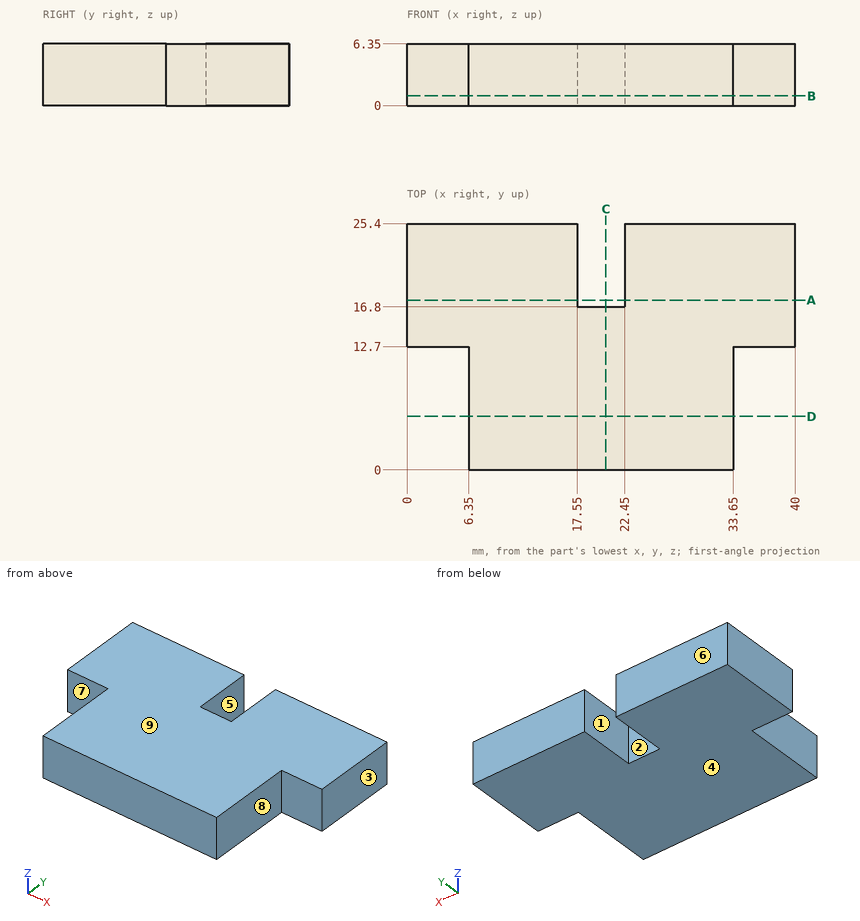
Part print with two shaded views. Sizes in mm from the minimum x, y, z corner. A direction names the side the tool comes from. Coordinates: 2 decimals unless noted, no trailing zeros. Order: outer loops, then holes, each group sorted by start corner. A loop starts at its lowest first (then second) coordinate and runs counter-clockwise, first axis right, second up. Notation, with made-up numbers: (-16, -4.75) - (2, -4.75) arc R20 ccw to (2, 22.25) - close; hole circle Ø1 at (31, 81). An arc over 180 degrees is marked (long way). Write item = value, one per line. Start each with the question number.
1) Saw through at A-A on y = 17.5. Write the cut outline in (x, z), then the cut area to 3 significant figures.
2) Wall check: line 1 along X through (y, z) = (19.75, 4.5); line 2 along Y through (x, z) = (6, 6.25); line 3 along X through (y, z) = (6, 3.5). Give the ranges that are in metal, low to high. Write a range as from..to.
3) Saw through at D-D on y = 5.5. Write the cut outline in (x, z).
4) Saw through at C-C on x = 20.5. Write the cut outline in (y, z).
5) Flat gauge pins, fed straight in: pin 1 Ø8 at (x, y) = (20.5, 19.5) entering from -Z; pin 2 Ø2.5 at (x, z) = (20.5, 4) entering from +Y; pin 3 Ø3 at (y, z) = (7, 2.5) entering from -X; pin 4 Ø1.9 at (x, z) = (35.5, 3) entering from -Y. Where does each tip first touch, or does it go through?
6) 3-axis set-ups, long thin cutter, end or side, ignore diameter. For the marked faces 5, 6, 7, 8 and 9: which of +Z, -Z, +X, -X, +Y, -Y reach the whole face in a straight line?
7) Two-plate mould, pull along X, no slides. Class the marked faces 1, 2, 3 and 4: pulls with the +X half, pulls with the -X half, needs draft (parallel to the pull), parting line crosses it, or undercut.
8) Saw through at B-B on z = 1. Write the cut outline in (x, y), then the cut area to 3 significant figures.
From the geometry:
q1.outline = (0, 0) - (17.55, 0) - (17.55, 6.35) - (0, 6.35) - close; (22.45, 0) - (40, 0) - (40, 6.35) - (22.45, 6.35) - close
q1.area = 223 mm^2
q2.line_1 = 0..17.55, 22.45..40
q2.line_2 = 12.7..25.4
q2.line_3 = 6.35..33.65
q3.outline = (6.35, 0) - (33.65, 0) - (33.65, 6.35) - (6.35, 6.35) - close
q4.outline = (0, 0) - (16.8, 0) - (16.8, 6.35) - (0, 6.35) - close
q5.pin_1 = 0
q5.pin_2 = 16.8
q5.pin_3 = 6.35
q5.pin_4 = 12.7
q6.face_5 = +Z, -Z, +Y
q6.face_6 = +Z, -Z, +X, -X, +Y
q6.face_7 = +Z, -Z, -X, -Y
q6.face_8 = +Z, -Z, +X, -Y
q6.face_9 = +Z, +X, -X, +Y, -Y
q7.face_1 = undercut
q7.face_2 = undercut
q7.face_3 = pulls with the +X half
q7.face_4 = needs draft
q8.outline = (0, 12.7) - (6.35, 12.7) - (6.35, 0) - (33.65, 0) - (33.65, 12.7) - (40, 12.7) - (40, 25.4) - (22.45, 25.4) - (22.45, 16.8) - (17.55, 16.8) - (17.55, 25.4) - (0, 25.4) - close
q8.area = 813 mm^2
